from build123d import *

# Parameters (mm, degrees)
SKETCH_W     = 83
SKETCH_H     = 83
PAD_DEPTH    = 16.5
FILLET_R     = 7.5
CHAMFER_SIZE = 1
PAD001_DEPTH = 19
FILLET001_R  = 1
SKETCH002_R  = 2
PAD002_DEPTH = 4
SKETCH003_R  = 1.7
PAD003_DEPTH = 6.5
SKETCH004_R  = 2
PAD004_DEPTH = 8
FILLET002_R  = 1.2
FILLET003_R  = 1.2
FILLET004_R  = 1
SKETCH005_R  = 2
PAD005_DEPTH = 15


with BuildPart() as part:
    # Sketch → Pad (new body, symmetric)
    with BuildSketch(Plane.XY):
        Rectangle(SKETCH_W, SKETCH_H)
    extrude(amount=PAD_DEPTH, both=True)

    # Fillet
    fillet_edges = [part.edges().sort_by_distance(p)[0] for p in [
        (41.5, -41.5, 0),
        (-41.5, -41.5, 0),
        (41.5, 41.5, 0),
        (-41.5, 41.5, 0),
    ]]
    fillet(fillet_edges, radius=FILLET_R)

    # Chamfer
    chamfer_edges = [part.edges().sort_by_distance(p)[0] for p in [
        (0, 41.5, 16.5),
        (-39.303301, 39.303301, 16.5),
        (-41.5, 0, 16.5),
        (41.5, 0, 16.5),
        (39.303301, 39.303301, 16.5),
        (-39.303301, -39.303301, 16.5),
        (0, -41.5, 16.5),
        (39.303301, -39.303301, 16.5),
        (39.303301, -39.303301, -16.5),
        (0, -41.5, -16.5),
        (-39.303301, -39.303301, -16.5),
        (-41.5, 0, -16.5),
        (41.5, 0, -16.5),
        (39.303301, 39.303301, -16.5),
        (0, 41.5, -16.5),
        (-39.303301, 39.303301, -16.5),
    ]]
    chamfer(chamfer_edges, length=CHAMFER_SIZE)

    # Sketch001 (on Face13 of Chamfer) → Pad001 (join)
    with BuildSketch(Plane.YZ.offset(41.5)):
        Polygon((18.5, 11), (18.5, -11), (25, -17.5), (31.5, -11), (31.5, 11), (25, 17.5), align=None)
    extrude(amount=PAD001_DEPTH)

    # Fillet001
    fillet001_edges = [part.edges().sort_by_distance(p)[0] for p in [
        (51, 31.5, 11),
        (51, 18.5, 11),
        (51, 25, 17.5),
        (51, 18.5, -11),
        (51, 25, -17.5),
        (51, 31.5, -11),
    ]]
    fillet(fillet001_edges, radius=FILLET001_R)

    # Sketch002 (on Face12 of Fillet001) → Pad002 (join)
    with BuildSketch(Plane.YZ.offset(60.5)):
        with Locations((25, 9.5)):
            Circle(SKETCH002_R)
        with Locations((25, -9.5)):
            Circle(SKETCH002_R)
    extrude(amount=PAD002_DEPTH)

    # Sketch003 (on Face43 of Pad002) → Pad003 (join)
    with BuildSketch(Plane.YZ.offset(64.5)):
        with Locations((25, 9.5)):
            Circle(SKETCH003_R)
        with Locations((25, -9.5)):
            Circle(SKETCH003_R)
    extrude(amount=PAD003_DEPTH)

    # Sketch004 (on Face50 of Pad003) → Pad004 (join)
    with BuildSketch(Plane.YZ.offset(71)):
        with Locations((25, 9.5)):
            Circle(SKETCH004_R)
        with Locations((25, -9.5)):
            Circle(SKETCH004_R)
    extrude(amount=PAD004_DEPTH)

    # Fillet002
    fillet002_edges = [part.edges().sort_by_distance(p)[0] for p in [
        (79, 23, 9.5),
    ]]
    fillet(fillet002_edges, radius=FILLET002_R)

    # Fillet003
    fillet003_edges = [part.edges().sort_by_distance(p)[0] for p in [
        (79, 23, -9.5),
    ]]
    fillet(fillet003_edges, radius=FILLET003_R)

    # Cone → Cone (revolve)
    with BuildSketch(Plane(origin=(-41.5, 0, 0), x_dir=(0, -1, 0), z_dir=(0, 0, -1))):
        Polygon((0, 0), (4, 0), (3, 15), (0, 15), align=None)
    revolve(axis=Axis((-41.5, 0, 0), (-1, 0, 0)))

    # Fillet004
    fillet004_edges = [part.edges().sort_by_distance(p)[0] for p in [
        (-56.5, 3, 0),
    ]]
    fillet(fillet004_edges, radius=FILLET004_R)

    # Sketch005 (on Face4 of Fillet004) → Pad005 (join)
    with BuildSketch(Plane(origin=(-56.5, 0, 0), x_dir=(0, -1, 0), z_dir=(-1, 0, 0))):
        Circle(SKETCH005_R)
    extrude(amount=PAD005_DEPTH)


solid = part.part
Work out the finished part from the listing and answer in its coordinate system (mm). A direction names the side the tool comes from. Give positions to 0.01 mm unless a question says otherwise; leave off trailing zeros. Loops run counter-clockwise (first coordinate to the right, second up) from the corner with the lowest first, then second, coordinate; pieces in that order, holes last. Notation, with made-up numbers: M 45.25,-21 L 49.25,-21 A13 ccw 49.25,-15 Z; hole C -40,67 d2. An arc over 180 degrees is marked long. Use CSV: the item, a comma, the result in double quotes.
1) Determine the mould class of faces 4 (the conical face through (38.771, -38.667, -16.326)), 5 (the flat face through (-41.5, 0, 7)), 6 (the flat face through (0, -41.5, 0)), 7 (the cylindrical face through (67.7, 26.57, -10.15)) for opening direction X: released by +X, released by -X, zero draft, split by the parting line, or undercut.
Answer:
face 4,"released by +X"
face 5,"released by -X"
face 6,"zero draft"
face 7,"undercut"
2) Consider L1, parallel to X at y = -11.5, z = -0.5; L2, parallel to Z at x = 37.5, y = -11.5; L3, parallel to X at y = 31, z = -4. Determine where each line is inside the solid, lowest interval first.
Answer:
L1,"-41.5 to 41.5"
L2,"-16.5 to 16.5"
L3,"-41.5 to 60.5"
3) Given P1, Ø0.8, axis at y = 25, z = 16, coming from the -X side; P2, Ø4, axis at y = -5.5, z = -7.5, coming from the -X side; P3, Ø2, axis at y = 18.5, z = 1, coming from the +X side, each flat-ended and moving along its own axis, determine where each tip first touches the part or whether it passes through.
Answer:
P1,"x = -41.4"
P2,"x = -41.5"
P3,"x = 60.5"
4) Find section C-C on x = 55. Write down the section's boundary in (y, z).
Answer:
outline,"M 18.5,-10.59 A1 ccw 18.79,-11.29 L 24.29,-16.79 A1 ccw 25.71,-16.79 L 31.21,-11.29 A1 ccw 31.5,-10.59 L 31.5,10.59 A1 ccw 31.21,11.29 L 25.71,16.79 A1 ccw 24.29,16.79 L 18.79,11.29 A1 ccw 18.5,10.59 Z"
5) Find section A-A on y = -9. Write down the section's boundary in (x, z).
Answer:
outline,"M -41.5,-15.5 L -40.5,-16.5 L 40.5,-16.5 L 41.5,-15.5 L 41.5,15.5 L 40.5,16.5 L -40.5,16.5 L -41.5,15.5 Z"
6) Which of the six approach directions +Z, -Z, +X, -X, +Y, -Y give full straight-line access (tool end or side, diameter ignored) to faces 1 (the flat face through (51, 18.5, 0)), 2 (the flat face through (50.9, 21.5, -14)), 3 (the conical face through (38.667, 38.771, -16.326))?
Answer:
face 1,"+Z, -Z, +X, -Y"
face 2,"-Z, +X, -Y"
face 3,"-Z, +X, +Y"
7) Find section B-B on z = 14. Write down the section's boundary in (x, y).
Answer:
outline,"M -41.5,-34 A7.5 ccw -34,-41.5 L 34,-41.5 A7.5 ccw 41.5,-34 L 41.5,21.5 L 60.5,21.5 L 60.5,28.5 L 41.5,28.5 L 41.5,34 A7.5 ccw 34,41.5 L -34,41.5 A7.5 ccw -41.5,34 Z"
